Input: part model. Units: mm. Frame: model coordinates. Face numbers are marked on the shaded views. A direction names the side the tool comes from. Round coordinates to 2 decimals unless told otherwise and drop trailing zeros. Order: outer loops, then holes, each group sorted by start corner. A loop starts at its lowest first (then second) coordinate and runs counter-clockwise, first axis right, second up. Notation, with made-up numbers: (87, 30.25) -> (144, 30.25) arc R21 ccw to (144, 50.25) -> close; hole circle Ø3 at (20, 17). An arc over 180 degrees is marked (long way). Use a Markdown table: item, result.
from build123d import *

# Parameters (mm, degrees)
F0_R     = 9.525
F1_DEPTH = 127
F2_R     = 9.525
F3_DEPTH = 34.798
F4_DEPTH = 22.86


with BuildPart() as f1:
    # F0 (on Front) → F1 (new body)
    with BuildSketch(Plane.XZ):
        Polygon((-10.003853, -26.378524), (9.046147, -26.378524), (9.046147, -13.678524), (18.571147, -13.678524), (18.571147, 37.121476), (-19.528853, 37.121476), (-19.528853, -13.678524), (-10.003853, -13.678524), align=None)
        with Locations((-0.478853, 11.721476)):
            Circle(F0_R, mode=Mode.SUBTRACT)
    extrude(amount=F1_DEPTH)

    # F2 (on Right) → F3 (cut)
    with BuildSketch(Plane.YZ):
        with Locations((-93.907245, 11.488916)):
            Circle(F2_R)
        with Locations((-31.356047, 11.658282)):
            Circle(F2_R)
    extrude(amount=-F3_DEPTH, mode=Mode.SUBTRACT)

    # F2 (on Right) → F4 (cut)
    with BuildSketch(Plane.YZ):
        with Locations((-93.907245, 11.488916)):
            Circle(F2_R)
        with Locations((-31.356047, 11.658282)):
            Circle(F2_R)
    extrude(amount=F4_DEPTH, mode=Mode.SUBTRACT)


solid = f1.part
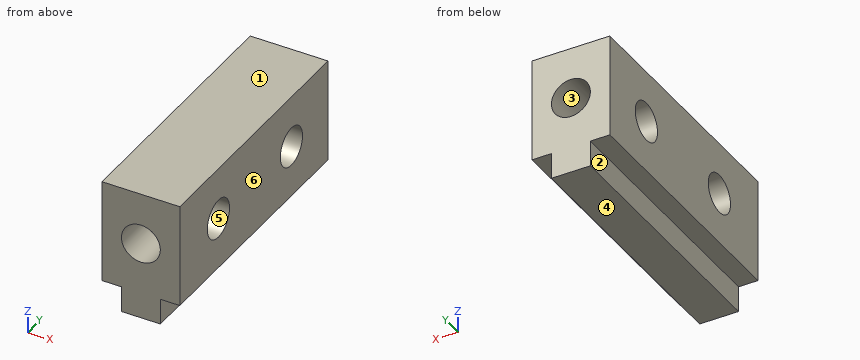
1) Pull-direction query (Z, two-part tool) for the marked faces 3, 4, 5 and 6; classes: +Z half, -Z half, draft (parallel to the pull), parting line (faces both ways), or undercut.
Results found:
| item | result |
|---|---|
| face 3 | undercut |
| face 4 | -Z half |
| face 5 | undercut |
| face 6 | draft |
2) Cut plane A-A on x = 3.5. Return loops of the section in (y, z) (3 decimals), and give its area (3 significant figures).
Results found:
| item | result |
|---|---|
| outline | (-127, -26.379) -> (0, -26.379) -> (0, 3.067) -> (-27.243, 3.067) arc R9.525 cw to (-35.47, 3.067) -> (-89.457, 3.067) arc R9.525 cw to (-98.357, 3.067) -> (-127, 3.067) -> close; (-127, 20.376) -> (-97.335, 20.376) arc R9.525 cw to (-90.479, 20.376) -> (-35.194, 20.376) arc R9.525 cw to (-27.518, 20.376) -> (0, 20.376) -> (0, 37.121) -> (-127, 37.121) -> close |
| area | 5,850 mm² |
3) Cut plane B-B on z = 13. Return loops of the section in (x, y).
Results found:
| item | result |
|---|---|
| outline | (-19.53, -127) -> (-9.92, -127) -> (-9.92, -103.31) -> (-19.53, -103.31) -> close; (-19.53, -84.5) -> (-9.92, -84.5) -> (-9.92, -40.79) -> (-19.53, -40.79) -> close; (-19.53, -21.93) -> (-9.92, -21.93) -> (-9.92, 0) -> (-19.53, 0) -> close; (8.96, -127) -> (18.57, -127) -> (18.57, -103.31) -> (8.96, -103.31) -> close; (8.96, -84.5) -> (18.57, -84.5) -> (18.57, -40.79) -> (8.96, -40.79) -> close; (8.96, -21.93) -> (18.57, -21.93) -> (18.57, 0) -> (8.96, 0) -> close |
4) Cut plane C-C on y = -24.5. Return loops of the section in (x, z) (3 decimals), and give its area (3 significant figures).
Results found:
| item | result |
|---|---|
| outline | (-19.529, -13.679) -> (-10.004, -13.679) -> (-10.004, -26.379) -> (9.046, -26.379) -> (9.046, -13.679) -> (18.571, -13.679) -> (18.571, 5.046) -> (6.316, 5.046) arc R9.525 cw to (-7.273, 5.046) -> (-19.529, 5.046) -> close; (-19.529, 18.27) -> (-7.395, 18.27) arc R9.525 cw to (6.438, 18.27) -> (18.571, 18.27) -> (18.571, 37.121) -> (-19.529, 37.121) -> close |
| area | 1,620 mm² |
5) Cut plane D-D on y = -66. Return loops of the section in (x, z) (3 decimals).
Results found:
| item | result |
|---|---|
| outline | (-19.529, -13.679) -> (-10.004, -13.679) -> (-10.004, -26.379) -> (9.046, -26.379) -> (9.046, -13.679) -> (18.571, -13.679) -> (18.571, 37.121) -> (-19.529, 37.121) -> close; hole circle Ø19.05 at (-0.479, 11.721) |
6) Line query: L1, parallel to Y at x = -17, z = 7.5; L2, parallel to Y at x = 12.5, z = 16; L3, parallel to Z at x = 15, y = -73. Output: solid intervals per line, ascending. Write a range as [from, to].
Results found:
| item | result |
|---|---|
| L1 | y = [-127, -102.56], [-85.26, -39.93], [-22.79, 0] |
| L2 | y = [-127, -102.3], [-85.52, -39.83], [-22.88, 0] |
| L3 | z = [-13.68, 37.12] |
7) Pin query (flat end, axial travel): pin 1 Ø10.5 at (x, y) = (15.5, -91) entering from -Z; pin 2 Ø6.5 at (y, z) = (-79.5, -22.5) entering from -X; pin 3 Ø14 at (y, z) = (-42, -21) entering from +X. Return the tip coordinate at first contact, or that it passes through.
Results found:
| item | result |
|---|---|
| pin 1 | stops at z = -13.68 |
| pin 2 | stops at x = -10 |
| pin 3 | stops at x = 9.05 |
8) Set-up query: the marked faces 1 and 2. Return all of +Z, -Z, +X, -X, +Y, -Y with unobstructed straight access to the full face (end or side cutting, diameter ignored); none if empty.
Results found:
| item | result |
|---|---|
| face 1 | +Z, +X, -X, +Y, -Y |
| face 2 | -Z, -X, +Y, -Y |
